The model under review builds one solid part; all positions refer to its coordinate system, in mm. A direction names the side the tool comes from. Coordinates: 2 decimals unless noted, no trailing zeros. Order: outer loops, then holes, each group sorted by start corner. A loop starts at its lowest first (then second) coordinate and runs counter-clockwise, first axis right, second up. Notation, with made-up numbers: M 53.5,-28.75 L 76.5,-28.75 A15 cw 76.5,-16.75 Z; hole C 4.25,13.25 d4. An arc over 180 degrees is marked long. Answer as CSV lines item,"result". Start each with the question number.
Q1. Consider section B-B on y = 35. State how many separate pieces and enclosed holes the cut face has, and give its area (3 significant figures).
Q2. For P1, Ø10, axis at x = 7.5, y = 30, coming from the +Z side; P2, Ø2, axis at x = -0.5, y = 7.5, coming from the +Z side; P3, Ø5, axis at x = -3.5, z = 0, coming from the +Y side, all flat-tipped, find the tip position at first contact; note any pin that passes through.
Q3. Wall thickness on L1, parallel to X at y = 28, z = 0; L2, parallel to X at y = 1, z = 0; L3, parallel to X at y = 35, z = 2.5: over which ranges is each line inside the solid? List them lowest first. Write a range as [from, to].
Q4. The part is to be moulded in two halves that separate along Z. For faces 4 (the face through (0, 1.5, 0)), 5 (the face through (1, 19, 0)), 6 (the face through (-5, 0, 3)), say which applies: +Z half, -Z half, draft (parallel to the pull), parting line (faces both ways), or undercut.
Q5. Consider section C-C on y = 20.5. Write out the cut boundary in (x, z).
Q6. Machinability: for faces 1 (the face through (-1.412, 19.248, -4.596)), 2 (the face through (0, 37.5, 0)), 3 (the face through (0, 32.5, 15)), which of the approach directions +Z, -Z, +X, -X, +Y, -Y give a long, thin tool a straight path to every point of the face, cutting with its end or side? Answer none if there is none.
from build123d import *

# Parameters (mm, degrees)
SKETCH1_R           = 12.5
SKETCH1_R_2         = 2
BOSS_EXTRUDE1_DEPTH = 42.5
SKETCH2_R           = 5.5
CUT_EXTRUDE1_DEPTH  = 1.5
BOSS_EXTRUDE3_START = -10
SKETCH3_R           = 35
SKETCH3_R_2         = 12.5
BOSS_EXTRUDE3_DEPTH = 10
SKETCH4_R           = 5
CUT_EXTRUDE5_DEPTH  = 10
CHAMFER7_SIZE       = 5
CUT_EXTRUDE6_START  = -5
SKETCH7_R           = 8
SKETCH7_R_2         = 5.5
SKETCH7_R_3         = 2
CUT_EXTRUDE6_DEPTH  = 5
CHAMFER8_SIZE       = 5


with BuildPart() as part:
    # Sketch1 → Boss-Extrude1 (new body)
    with BuildSketch(Plane(origin=(0, 0, 0), x_dir=(1, 0, 0), z_dir=(0, 1, 0))):
        with Locations(Location((0, 0, 0), (0, 0, 270))):
            Circle(SKETCH1_R)
        with Locations(Location((3, 0, 0), (0, 0, 270))):
            Circle(SKETCH1_R_2, mode=Mode.SUBTRACT)
        with Locations(Location((-1.5, -2.598076211, 0), (0, 0, 270))):
            Circle(SKETCH1_R_2, mode=Mode.SUBTRACT)
        with Locations(Location((-1.5, 2.598076211, 0), (0, 0, 270))):
            Circle(SKETCH1_R_2, mode=Mode.SUBTRACT)
    extrude(amount=BOSS_EXTRUDE1_DEPTH)

    # Sketch2 → Cut-Extrude1 (cut)
    with BuildSketch(Plane.XZ):
        with Locations(Location((0, 0, 0), (0, 0, 270))):
            Circle(SKETCH2_R)
    extrude(amount=-CUT_EXTRUDE1_DEPTH, mode=Mode.SUBTRACT)

    # Sketch3 → Boss-Extrude3 (add)
    with BuildSketch(Plane(origin=(0, 42.5, 0), x_dir=(1, 0, 0), z_dir=(0, 1, 0)).offset(BOSS_EXTRUDE3_START)):
        with Locations(Location((0, 0, 0), (0, 0, 270))):
            Circle(SKETCH3_R)
        with Locations(Location((0, 0, 0), (0, 0, 270))):
            Circle(SKETCH3_R_2, mode=Mode.SUBTRACT)
    extrude(amount=BOSS_EXTRUDE3_DEPTH)

    # Sketch4 → Cut-Extrude5 (cut)
    with BuildSketch(Plane(origin=(0, 42.5, 0), x_dir=(1, 0, 0), z_dir=(0, 1, 0))):
        with Locations(Location((-23, 0, 0), (0, 0, 270))):
            Circle(SKETCH4_R)
        with Locations(Location((-11.5, 19.918584287, 0), (0, 0, 270))):
            Circle(SKETCH4_R)
        with Locations(Location((11.5, 19.918584287, 0), (0, 0, 270))):
            Circle(SKETCH4_R)
        with Locations(Location((23, 0, 0), (0, 0, 270))):
            Circle(SKETCH4_R)
        with Locations(Location((11.5, -19.918584287, 0), (0, 0, 270))):
            Circle(SKETCH4_R)
        with Locations(Location((-11.5, -19.918584287, 0), (0, 0, 270))):
            Circle(SKETCH4_R)
    extrude(amount=-CUT_EXTRUDE5_DEPTH, mode=Mode.SUBTRACT)

    # Chamfer7
    chamfer7_edges = [part.edges().sort_by_distance(p)[0] for p in [
        (-23, 32.5, -5),
        (-23, 42.5, -5),
        (-11.5, 32.5, 14.918584287),
        (-11.5, 42.5, 14.918584287),
        (11.5, 32.5, 14.918584287),
        (11.5, 42.5, 14.918584287),
        (23, 32.5, -5),
        (23, 42.5, -5),
        (11.5, 32.5, -24.918584287),
        (11.5, 42.5, -24.918584287),
        (-11.5, 32.5, -24.918584287),
        (-11.5, 42.5, -24.918584287),
    ]]
    chamfer(chamfer7_edges, length=CHAMFER7_SIZE - 0.0001)  # a hair under: the kernel refuses the full size

    # Sketch7 → Cut-Extrude6 (cut)
    # profile 1 of 2: a face of its own
    with BuildSketch(Plane(origin=(0, 42.5, 0), x_dir=(1, 0, 0), z_dir=(0, 1, 0)).offset(CUT_EXTRUDE6_START)):
        with Locations(Location((0, 0, 0), (0, 0, 270))):
            Circle(SKETCH7_R)
        with Locations(Location((0, 0, 0), (0, 0, 90))):
            Circle(SKETCH7_R_2, mode=Mode.SUBTRACT)
    # profile 2 of 2: a face of its own
    with BuildSketch(Plane(origin=(0, 42.5, 0), x_dir=(1, 0, 0), z_dir=(0, 1, 0)).offset(CUT_EXTRUDE6_START)):
        with Locations(Location((0, 0, 0), (0, 0, 90))):
            Circle(SKETCH7_R_2)
        with Locations(Location((-1.5, 2.598076211, 0), (0, 0, 90))):
            Circle(SKETCH7_R_3, mode=Mode.SUBTRACT)
        with Locations(Location((-1.5, -2.598076211, 0), (0, 0, 90))):
            Circle(SKETCH7_R_3, mode=Mode.SUBTRACT)
        with Locations(Location((3, 0, 0), (0, 0, 90))):
            Circle(SKETCH7_R_3, mode=Mode.SUBTRACT)
    extrude(amount=CUT_EXTRUDE6_DEPTH, mode=Mode.SUBTRACT)

    # Chamfer8
    chamfer8_edges = [part.edges().sort_by_distance(p)[0] for p in [
        (0, 42.5, -8),
    ]]
    chamfer(chamfer8_edges, length=CHAMFER8_SIZE - 0.0001)  # a hair under: the kernel refuses the full size


solid = part.part
Evaluation:
1,separate pieces,"1"
1,enclosed holes,"9"
1,area,"2,750 mm²"
2,P1,"stops at z = 34.86"
2,P2,"stops at z = 12.5"
2,P3,"stops at y = 37.5"
3,L1,"x = [-12.5, 1], [5, 12.5]"
3,L2,"x = [-12.5, -5.5], [5.5, 12.5]"
3,L3,"x = [-34.91, -30.07], [-15.93, -3.5], [0.5, 15.93], [30.07, 34.91]"
4,face 4,"undercut"
4,face 5,"undercut"
4,face 6,"draft"
5,outline,"C 0,0 d25; hole C -1.5,-2.6 d4; hole C -1.5,2.6 d4; hole C 3,0 d4"
6,face 1,"+Y, -Y"
6,face 2,"+Y"
6,face 3,"-Y"
